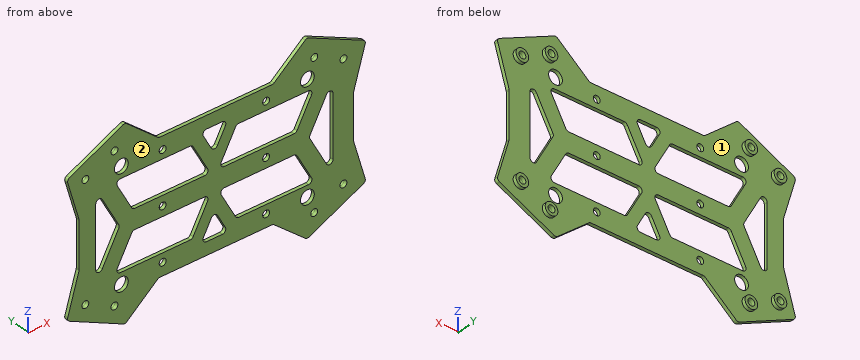
```python
from build123d import *

# Parameters (mm, degrees)
SKETCH1_R               = 1.5
BOSS_EXTRUDE1_DEPTH     = 1.5
CUT_EXTRUDE3_DEPTH      = 78.112196707
CUT_EXTRUDE3_DEPTH_BACK = 1.5
SKETCH2_R               = 3
SKETCH2_R_2             = 1.5
FILLET1_R               = 1.5
FILLET2_R               = 1.5
FILLET3_R               = 1.5
FILLET4_R               = 1.5
SKETCH3_R               = 2.75
SKETCH3_R_2             = 1.5
BOSS_EXTRUDE2_DEPTH     = 1.5


with BuildPart() as part:
    # Sketch1 → Boss-Extrude1 (new body)
    with BuildSketch(Plane(origin=(0, 0, 0), x_dir=(1, 0, 0), z_dir=(0, 1, 0))):
        with BuildLine():
            Line((-39.718703085, 39.786008686), (-64.143839052, 28.145904827))
            Line((-64.143839052, 28.145904827), (-58.793839052, 10))
            Line((-58.793839052, 10), (-58.793839052, 0))
            Line((-58.793839052, 0), (60.6, 0))
            Line((60.6, 0), (60.6, 10))
            Line((60.6, 10), (65.947243643, 28.142062598))
            Line((65.947243643, 28.142062598), (41.112235129, 39.795412747))
            ThreePointArc((41.112235129, 39.795412747), (40.285063102, 39.92539514), (39.517091476, 39.591735783))
            Line((39.517091476, 39.591735783), (25.966587834, 28.345739563))
            ThreePointArc((25.966587834, 28.345739563), (25.517849862, 28.089079971), (25.008630192, 28))
            Line((25.008630192, 28), (-23.705783083, 28))
            ThreePointArc((-23.705783083, 28), (-24.217369993, 28.089936585), (-24.667609729, 28.348961555))
            Line((-24.667609729, 28.348961555), (-38.111565458, 39.582951958))
            ThreePointArc((-38.111565458, 39.582951958), (-38.885366706, 39.920082337), (-39.718703085, 39.786008686))
        make_face()
        with Locations(Location((-43.45, 31, 0), (0, 0, 270))):
            Circle(SKETCH1_R, mode=Mode.SUBTRACT)
        with Locations(Location((-56.13, 25, 0), (0, 0, 270))):
            Circle(SKETCH1_R, mode=Mode.SUBTRACT)
        with Locations(Location((56.13, 25, 0), (0, 0, 270))):
            Circle(SKETCH1_R, mode=Mode.SUBTRACT)
        with Locations(Location((43.45, 31, 0), (0, 0, 270))):
            Circle(SKETCH1_R, mode=Mode.SUBTRACT)
    extrude(amount=BOSS_EXTRUDE1_DEPTH)

    # Sketch2 → Cut-Extrude3 (cut, two sides: drawn at the far end of the back side and taken through both)
    with BuildSketch(Plane(origin=(0, 0, 0), x_dir=(1, 0, 0), z_dir=(0, 1, 0)).offset(-CUT_EXTRUDE3_DEPTH_BACK)):
        with Locations(Location((40.45, 23.6, 0), (0, 0, 270))):
            Circle(SKETCH2_R)
        with Locations(Location((-40.45, 23.6, 0), (0, 0, 270))):
            Circle(SKETCH2_R)
        with Locations(Location((-22.5, 22.5, 0), (0, 0, 270))):
            Circle(SKETCH2_R_2)
        with Locations(Location((22.5, 22.5, 0), (0, 0, 270))):
            Circle(SKETCH2_R_2)
        Polygon((-6, 22.5), (6, 22.5), (0, 11.5), align=None)
        Polygon((1.740892766, 4.25), (9.649983676, 18.75), (43.45, 18.75), (35.540909091, 4.25), align=None)
        Polygon((-43.45, 18.75), (-35.540909091, 4.25), (-1.740892766, 4.25), (-9.649983676, 18.75), align=None)
        Polygon((41.196340782, 0), (51.6, 19.073375233), (51.6, 0), align=None)
        Polygon((-51.6, 0), (-41.196340782, 0), (-51.6, 19.073375233), align=None)
        with BuildLine():
            Line((21, 0), (24, 0))
            ThreePointArc((24, 0), (22.5, 1.5), (21, 0))
        make_face()
        with BuildLine():
            Line((-24, 0), (-21, 0))
            ThreePointArc((-21, 0), (-22.5, 1.5), (-24, 0))
        make_face()
    extrude(amount=CUT_EXTRUDE3_DEPTH + CUT_EXTRUDE3_DEPTH_BACK, mode=Mode.SUBTRACT)

    # Mirror1: part across plane


with BuildPart() as part_1:
    add(part.part)
    add(part.part.mirror(Plane.XY))

    # Fillet1
    fillet1_edges = [part_1.edges().sort_by_distance(p)[0] for p in [
        (1.740892766, 0.75, -4.25),
        (35.540909091, 0.75, -4.25),
        (43.45, 0.75, -18.75),
        (9.649983676, 0.75, -18.75),
        (1.740892766, 0.75, 4.25),
        (35.540909091, 0.75, 4.25),
        (43.45, 0.75, 18.75),
        (9.649983676, 0.75, 18.75),
        (-9.649983676, 0.75, 18.75),
        (-43.45, 0.75, 18.75),
        (-35.540909091, 0.75, 4.25),
        (-1.740892766, 0.75, 4.25),
        (-9.649983676, 0.75, -18.75),
        (-43.45, 0.75, -18.75),
        (-35.540909091, 0.75, -4.25),
        (-1.740892766, 0.75, -4.25),
    ]]
    fillet(fillet1_edges, radius=FILLET1_R)

    # Fillet2
    fillet2_edges = [part_1.edges().sort_by_distance(p)[0] for p in [
        (51.6, 0.75, -19.073375233),
        (-51.6, 0.75, -19.073375233),
        (41.196340782, 0.75, 0),
        (-51.6, 0.75, 19.073375233),
        (-41.196340782, 0.75, 0),
        (51.6, 0.75, 19.073375233),
    ]]
    fillet(fillet2_edges, radius=FILLET2_R)

    # Fillet3
    fillet3_edges = [part_1.edges().sort_by_distance(p)[0] for p in [
        (-6, 0.75, -22.5),
        (0, 0.75, -11.5),
        (6, 0.75, -22.5),
        (-6, 0.75, 22.5),
        (0, 0.75, 11.5),
        (6, 0.75, 22.5),
    ]]
    fillet(fillet3_edges, radius=FILLET3_R)

    # Fillet4
    fillet4_edges = [part_1.edges().sort_by_distance(p)[0] for p in [
        (-58.793839052, 0.75, 10),
        (60.6, 0.75, 10),
        (65.947243643, 0.75, 28.142062598),
        (-64.143839052, 0.75, 28.145904827),
        (-64.143839052, 0.75, -28.145904827),
        (65.947243643, 0.75, -28.142062598),
        (60.6, 0.75, -10),
        (-58.793839052, 0.75, -10),
    ]]
    fillet(fillet4_edges, radius=FILLET4_R)

    # Sketch3 → Boss-Extrude2 (add)
    # profile 1 of 4: a face of its own
    with BuildSketch(Plane(origin=(0, 1.5, 0), x_dir=(1, 0, 0), z_dir=(0, 1, 0))):
        with Locations(Location((-56.13, 25, 0), (0, 0, 270))):
            Circle(SKETCH3_R)
        with Locations(Location((-56.13, 25, 0), (0, 0, 270))):
            Circle(SKETCH3_R_2, mode=Mode.SUBTRACT)
    # profile 2 of 4: a face of its own
    with BuildSketch(Plane(origin=(0, 1.5, 0), x_dir=(1, 0, 0), z_dir=(0, 1, 0))):
        with Locations(Location((-43.45, 31, 0), (0, 0, 270))):
            Circle(SKETCH3_R)
        with Locations(Location((-43.45, 31, 0), (0, 0, 270))):
            Circle(SKETCH3_R_2, mode=Mode.SUBTRACT)
    # profile 3 of 4: a face of its own
    with BuildSketch(Plane(origin=(0, 1.5, 0), x_dir=(1, 0, 0), z_dir=(0, 1, 0))):
        with Locations(Location((43.45, 31, 0), (0, 0, 270))):
            Circle(SKETCH3_R)
        with Locations(Location((43.45, 31, 0), (0, 0, 270))):
            Circle(SKETCH3_R_2, mode=Mode.SUBTRACT)
    # profile 4 of 4: a face of its own
    with BuildSketch(Plane(origin=(0, 1.5, 0), x_dir=(1, 0, 0), z_dir=(0, 1, 0))):
        with Locations(Location((56.13, 25, 0), (0, 0, 270))):
            Circle(SKETCH3_R)
        with Locations(Location((56.13, 25, 0), (0, 0, 270))):
            Circle(SKETCH3_R_2, mode=Mode.SUBTRACT)
    boss_extrude2 = extrude(amount=BOSS_EXTRUDE2_DEPTH)

    # Mirror2: Boss-Extrude2 across plane
    add(boss_extrude2.mirror(Plane.XY))


solid = part_1.part
```
Source: CAD feature listing. Evaluate the final solid. Frame: model axes, mm. Face numbers are marked on the shaded views. Give positions to 0.01 mm unless a question says otherwise; leave off trailing zeros. Write each loop counter-clockwise with the first axis right and the second up, starting at its lowest first coordinate (ties: lowest second). Pieces come first, ordered by that corner, then holes.
1. Section query C-C (z = 31). Return the cut outline in (x, y), then the cut area to 3 significant figures.
2. Pull-direction query (X, two-part tool) for the marked faces 1 and 2; classes: +X half, -X half, draft (parallel to the pull), parting line (faces both ways), or undercut.
3. Material intervals for line 1 along Z through (x, y) = (16, 1.3); line 2 along X through (y, z) = (0.85, -31); line 3 along X through (y, z) = (2.3, 25), sorted ascending.
4. Section query B-B (x = 19). Return the cut outline in (y, z).
5. Section query A-A (y = 2.4). Count the separate pieces of the cut face and the enclosed holes in it, then the cut area to 3 significant figures.
6. First-contact query: pin 1 (1.6 mm diameter, centred on y = 0.5, z = 4, fed in from +X); pin 2 (0.8 mm diameter, centred on y = 1, z = 1, fed in from -X); pin 3 (10 mm diameter, centred on x = 10, z = -27.5, fed in from +Y). Flat tips, straight axial feed; report the tip coordinate or a pass-through.
7. Section query D-D (x = -56.13). Return the cut outline in (y, z) (3 decimals).
Output values:
1. outline: (-58.15, 0) - (-44.95, 0) - (-44.95, 3) - (-46.2, 3) - (-46.2, 1.5) - (-58.15, 1.5) - close; (-41.95, 0) - (-27.84, 0) - (-27.84, 1.5) - (-40.7, 1.5) - (-40.7, 3) - (-41.95, 3) - close; (29.16, 0) - (41.95, 0) - (41.95, 3) - (40.7, 3) - (40.7, 1.5) - (29.16, 1.5) - close; (44.95, 0) - (59.86, 0) - (59.86, 1.5) - (46.2, 1.5) - (46.2, 3) - (44.95, 3) - close
1. area: 90.0 mm2
2. face 1: undercut
2. face 2: draft
3. line 1: z = -28 to -18.75, -4.25 to 4.25, 18.75 to 28
3. line 2: x = -58.15 to -44.95, -41.95 to -27.84, 29.16 to 41.95, 44.95 to 59.86
3. line 3: x = -58.88 to -57.63, -54.63 to -53.38, 53.38 to 54.63, 57.63 to 58.88
4. outline: (0, -28) - (1.5, -28) - (1.5, -18.75) - (0, -18.75) - close; (0, -4.25) - (1.5, -4.25) - (1.5, 4.25) - (0, 4.25) - close; (0, 18.75) - (1.5, 18.75) - (1.5, 28) - (0, 28) - close
5. separate pieces: 8
5. enclosed holes: 8
5. area: 134 mm2
6. pin 1: stops at x = 60.6
6. pin 2: stops at x = -58.79
6. pin 3: stops at y = 1.5
7. outline: (0, -31.965) - (1.5, -31.965) - (1.5, -27.75) - (3, -27.75) - (3, -26.5) - (0, -26.5) - close; (0, -23.5) - (3, -23.5) - (3, -22.25) - (1.5, -22.25) - (1.5, 22.25) - (3, 22.25) - (3, 23.5) - (0, 23.5) - close; (0, 26.5) - (3, 26.5) - (3, 27.75) - (1.5, 27.75) - (1.5, 31.965) - (0, 31.965) - close
